Build history of the part. All positions in model axes, mm. Face numbers are marked on the shaded views. A direction names the side the tool comes from. Coordinates: 2 decimals unless noted, no trailing zeros. Loops run counter-clockwise (first coordinate to the right, second up) from the corner with the lowest first, then second, coordinate; pieces in that order, holes last.
Item 1: Flat gauge pins, fed straight in: pin 1 (1.5 mm diameter, centred on x = -2.5, z = 19.5, fed in from -Y); pin 2 (12 mm diameter, centred on y = -8.5, z = 18, fed in from -X); pin 3 (4 mm diameter, centred on x = -6, z = 2.5, fed in from +Y). Where does each tip first touch, or does it go through?
Item 2: Drill centre lines: line 1 along Y through (x, z) = (0, 9.5); line 2 along Z through (x, y) = (8, 1.25); line 3 along Z through (x, y) = (8.25, 12.25). Where is each one in solid material? Low to high.
Item 3: Cut at C-C (z = 19.5). List the corners of the cut face in (x, y) (3 decimals), and give its area (3 significant figures).
Item 4: Cut at A-A (x = 0). List the corners of the cut face in (y, z) (3 decimals), and give its area (3 significant figures).
Item 5: 3-axis set-ups, long thin cutter, end or side, ignore diameter. For the marked faces 4, 5 and 6: which of +Z, -Z, +X, -X, +Y, -Y reach the whole face in a straight line?
Item 6: Mould opens along Y. For the marked faces 1, 2 and 3 say: released by +Y, released by -Y, zero draft, split by the parting line, or undercut.
Item 7: Cut at D-D (z = 1.75). List the corners of the cut face in (x, y).
from build123d import *

# Parameters (mm, degrees)
F2_SIZE2       = 10
F2_SIZE        = 2
F4_D           = 8.8
F4_CBORE_D     = 14.25
F4_CBORE_DEPTH = 8


with BuildPart() as f1:
    # F0 (on Front) → F1 (revolve)
    with BuildSketch(Plane.XZ):
        Polygon((-15, 0), (0, 0), (0, 24), (-13.5, 24), (-13.5, 8), (-7, 8), (-7, 4), (-15, 4), align=None)
    revolve(axis=Axis((0, 0, 12), (0, 0, -1)))

    # F2
    f2_edges = [f1.edges().sort_by_distance(p)[0] for p in [
        (13.5, 0, 24),
    ]]
    chamfer(f2_edges, length=F2_SIZE, length2=F2_SIZE2)

    # F4 (through all)
    with Locations(Plane.XY.offset(24)):
        with Locations((0, 0)):
            CounterBoreHole(F4_D / 2, F4_CBORE_D / 2, F4_CBORE_DEPTH)


solid = f1.part
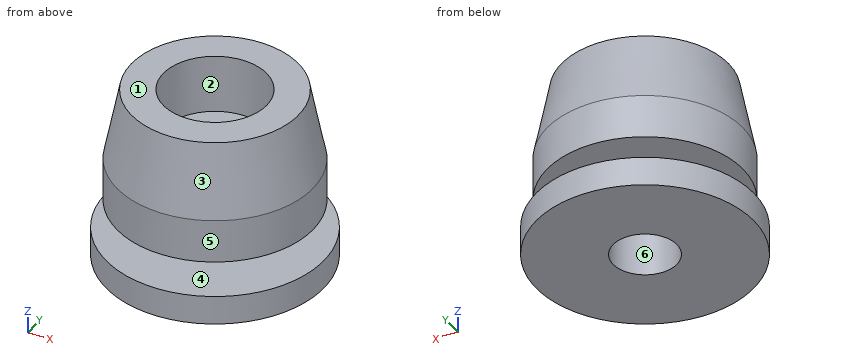
Filled sheet:
1. pin 1: stops at y = -12.35
1. pin 2: stops at x = -12.9
1. pin 3: stops at y = 14.46
2. line 1: y = -13.5 to -4.4, 4.4 to 13.5
2. line 2: z = 0 to 4, 8 to 24
2. line 3: z = 0 to 4
3. outline: circle Ø24.8 at (0, 0); hole circle Ø14.25 at (0, 0)
3. area: 324 mm2
4. outline: (-15, 0) - (-4.4, 0) - (-4.4, 16) - (-7.125, 16) - (-7.125, 24) - (-11.5, 24) - (-13.5, 14) - (-13.5, 8) - (-7, 8) - (-7, 4) - (-15, 4) - close; (4.4, 0) - (15, 0) - (15, 4) - (7, 4) - (7, 8) - (13.5, 8) - (13.5, 14) - (11.5, 24) - (7.125, 24) - (7.125, 16) - (4.4, 16) - close
4. area: 333 mm2
5. face 4: none
5. face 5: +Z
5. face 6: +Z, -Z
6. face 1: zero draft
6. face 2: undercut
6. face 3: split by the parting line
7. outline: circle Ø30 at (0, 0); hole circle Ø8.8 at (0, 0)
